```python
from build123d import *

# Parameters (mm, degrees)
BOSS_EXTRUDE1_DEPTH = 3.5
SKETCH1_3_R         = 3.259306638
BOSS_EXTRUDE2_DEPTH = 1
SKETCH1_4_R         = 3.259306638
BOSS_EXTRUDE3_DEPTH = 15
FILLET1_R           = 0.4


with BuildPart() as part:
    # Sketch1 → Boss-Extrude1 (new body)
    with BuildSketch(Plane.ZY.offset(-9.072873839)):
        with BuildLine():
            Line((-22.564889637, -14.994040891), (-21.564889637, -14.994040891))
            Line((-21.564889637, -14.994040891), (-21.564889637, -15.574172475))
            ThreePointArc((-21.564889637, -15.574172475), (-20.933518787, -15.962670041), (-20.545021222, -16.594040891))
            Line((-20.545021222, -16.594040891), (-19.964889637, -16.594040891))
            Line((-19.964889637, -16.594040891), (-19.964889637, -17.594040891))
            Line((-19.964889637, -17.594040891), (-20.545021222, -17.594040891))
            ThreePointArc((-20.545021222, -17.594040891), (-20.933518787, -18.225411741), (-21.564889637, -18.613909306))
            Line((-21.564889637, -18.613909306), (-21.564889637, -19.194040891))
            Line((-21.564889637, -19.194040891), (-22.564889637, -19.194040891))
            Line((-22.564889637, -19.194040891), (-22.564889637, -18.613909306))
            ThreePointArc((-22.564889637, -18.613909306), (-23.196260487, -18.225411741), (-23.584758053, -17.594040891))
            Line((-23.584758053, -17.594040891), (-24.164889637, -17.594040891))
            Line((-24.164889637, -17.594040891), (-24.164889637, -16.594040891))
            Line((-24.164889637, -16.594040891), (-23.584758053, -16.594040891))
            ThreePointArc((-23.584758053, -16.594040891), (-23.196260487, -15.962670041), (-22.564889637, -15.574172475))
            Line((-22.564889637, -15.574172475), (-22.564889637, -14.994040891))
        make_face()
    extrude(amount=-BOSS_EXTRUDE1_DEPTH)

    # Sketch1_3 → Boss-Extrude2 (add)
    with BuildSketch(Plane.ZY.offset(-9.072873839)):
        with Locations(Location((-22.064889637, -17.094040891, 0), (0, 0, 270))):
            Circle(SKETCH1_3_R)
    extrude(amount=BOSS_EXTRUDE2_DEPTH)

    # Sketch1_4 → Boss-Extrude3 (add)
    with BuildSketch(Plane.ZY.offset(-9.072873839)):
        with Locations((-22.064889637, -17.094040891)):
            Circle(SKETCH1_4_R)
        with BuildLine():
            ThreePointArc((-23.752066801, -19.072280821), (-21.868548232, -14.501464942), (-20.694879361, -19.303808263))
            Line((-20.694879361, -19.303808263), (-23.752066801, -19.072280821))
        make_face(mode=Mode.SUBTRACT)
    extrude(amount=BOSS_EXTRUDE3_DEPTH)

    # Fillet1
    fillet1_edges = [part.edges().sort_by_distance(p)[0] for p in [
        (9.072873839, -16.594040891, -20.25495543),
        (9.072873839, -15.962670041, -20.933518787),
        (9.072873839, -15.284106683, -21.564889637),
        (9.072873839, -14.994040891, -22.064889637),
        (9.072873839, -15.284106683, -22.564889637),
        (9.072873839, -15.962670041, -23.196260487),
        (9.072873839, -16.594040891, -23.874823845),
        (9.072873839, -17.094040891, -24.164889637),
        (9.072873839, -17.594040891, -23.874823845),
        (9.072873839, -18.225411741, -23.196260487),
        (9.072873839, -18.903975098, -22.564889637),
        (9.072873839, -19.194040891, -22.064889637),
        (9.072873839, -18.903975098, -21.564889637),
        (9.072873839, -18.225411741, -20.933518787),
        (9.072873839, -17.594040891, -20.25495543),
        (9.072873839, -17.094040891, -19.964889637),
        (9.072873839, -13.834734253, -22.064889637),
    ]]
    fillet(fillet1_edges, radius=FILLET1_R)


solid = part.part
```
Source: CAD feature listing. Evaluate the final solid. Frame: model axes, mm. A direction names the side the tool comes from. Give positions to 0.01 mm unless a question says otherwise; leave off trailing zeros. Write each loop counter-clockwise with the first axis right and the second up, starting at its lowest first coordinate (ties: lowest second). Pieces come first, ordered by that corner, then holes. Notation, with made-up numbers: (-28, 61) - (22, 61) arc R19 ccw to (22, 81) - close; hole circle Ø6 at (5.5, 76). An arc over 180 degrees is marked (long way). One line per item, written item: value. Start each with the question number.
Q1. Section query A-A, the plane x = 11.5. Return the cut outline in (y, z).
Q2. Section query C-C, the plane x = 8.25. Return the cut outline in (y, z), then the cut area to 3 significant figures.
Q3. Set-up query: faces 1 (the face through (11, -18.22, -20.93)), 2 (the face through (11, -14.994, -22)), 3 (the face through (11, -16, -20.9)). Return all of +Z, -Z, +X, -X, +Y, -Y with unobstructed straight access to the full face (end or side cutting, diameter ignored); none if empty.
Q4. Section query B-B, the plane x = 0.75. Return the cut outline in (y, z), then the cut area to 3 significant figures.
Q5. First-contact query: pin 1 Ø0.5 at (x, z) = (10.5, -24) entering from -Y; pin 2 Ø2 at (x, z) = (-4, -23.5) entering from -Y; pin 3 Ø0.5 at (x, y) = (11, -15.5) entering from +Z. Flat tips, straight axial feed; report the tip coordinate or a pass-through.
Q6. Material intervals for probe 1 along Y at (x, z) = (-0.5, -22); probe 2 along Z at (x, y) = (-4.5, -17); probe 3 along X at (y, z) = (-17.75, -22.5), sorted ascending. Write a range as from..to.
Q7. Draft query along Z for faces 4 (the face through (1.17, -19.19, -22.2)), 5 (the face through (-5.927, -19.3, -22.8)), 6 (the face through (11, -17, -19.965)). Return one class per face: +Z half, -Z half, draft (parallel to the pull), parting line (faces both ways), or undercut.
Answer:
1. outline: (-19.19, -22.56) - (-18.61, -22.56) arc R1.6 ccw to (-17.59, -23.58) - (-17.59, -24.16) - (-16.59, -24.16) - (-16.59, -23.58) arc R1.6 ccw to (-15.57, -22.56) - (-14.99, -22.56) - (-14.99, -21.56) - (-15.57, -21.56) arc R1.6 ccw to (-16.59, -20.55) - (-16.59, -19.96) - (-17.59, -19.96) - (-17.59, -20.55) arc R1.6 ccw to (-18.61, -21.56) - (-19.19, -21.56) - close
2. outline: circle Ø6.52 at (-17.09, -22.06)
2. area: 33.4 mm2
3. face 1: +Z, +X, -Y
3. face 2: +Z, -Z, +X, +Y
3. face 3: +Z, +X, +Y
4. outline: circle Ø6.52 at (-17.09, -22.06); hole (-19.3, -20.69) - (-19.07, -23.75) arc R2.6 ccw (long way) to start
4. area: 13.2 mm2
5. pin 1: stops at y = -17.59
5. pin 2: stops at y = -20.32
5. pin 3: stops at z = -21.2
6. probe 1: y = -20.35..-19.2, -14.49..-13.84
6. probe 2: z = -25.32..-24.66, -19.47..-18.81
6. probe 3: x = 8.07..12.57
7. face 4: undercut
7. face 5: draft
7. face 6: +Z half
